Geometry check sheet. Reference: the model listing, model coordinates, mm. A direction names the side the tool comes from. Give positions to 0.01 mm unless a question says otherwise; leave off trailing zeros. Loops run counter-clockwise (first coordinate to the right, second up) from the corner with the lowest first, then second, coordinate; pieces in that order, holes last.
1. Tool access check on faces 4 (the cylindrical face through (28.276, 121.639, -3.057)), 5 (the flat face through (3.019, 170, -3)), 6 (the flat face through (14.548, 114.345, -3.057)). Record the directions out of +Z, -Z, +X, -X, +Y, -Y that give a thin tool (end or side, any length) a straight path to the whole face; none if there is none.
2. Cross-section at D-D, the plane y = 134. Record the cut outline in (x, z), plus the area to 3 significant figures.
3. Cross-section at A-A, the plane z = -4.75. Record the cut outline in (x, y).
4. Cross-section at B-B, the plane x = 18. Record the cut outline in (y, z).
5. Material ranges on L1, parallel to Y at x = 19.75, z = -4; L2, parallel to X at y = 184, z = -4.5; L3, parallel to Y at x = 6, z = -4, recorded low to high.
6. Go/stop test with flat-tipped pins: pin 1 Ø3 at (y, z) = (96, -3) entering from -X; pin 2 Ø1.9 at (y, z) = (171.5, -4) entering from +X. Record where each tip stops, or that it passes through.
7. Cross-section at C-C, the plane y = 95.5. Record the cut outline in (x, z).
8. Release check for a two-part mould opening along Y. For faces 1 (the flat face through (15.196, 113.191, -3.057)), 2 (the cylindrical face through (2.642, 133.722, -3.057)), 3 (the flat face through (3.019, 93, -3)) record: +Y half, -Y half, draft (parallel to the pull), parting line (faces both ways), or undercut.
from build123d import *

# Parameters (mm, degrees)
BOSS_EXTRUDE1_DEPTH = 6.2
SKETCH2_W           = 22.942955783
SKETCH2_H           = 33.63345143
CUT_EXTRUDE1_DEPTH  = 10
SKETCH3_W           = 6.2
SKETCH3_H           = 21.335576668
CUT_EXTRUDE2_DEPTH  = 10
SKETCH4_W           = 6.2
SKETCH4_H           = 34.092468675
CUT_EXTRUDE3_DEPTH  = 10


with BuildPart() as part:
    # Sketch1 → Boss-Extrude1 (new body)
    with BuildSketch(Plane.XY):
        with BuildLine():
            Line((5.938584497, 132.670572888), (23.853053602, 126.575547243))
            ThreePointArc((23.853053602, 126.575547243), (28.280634989, 121.537232872), (24.198169049, 116.215432378))
            Line((24.198169049, 116.215432378), (5.937692527, 110.081409755))
            ThreePointArc((5.937692527, 110.081409755), (3.69123593, 108.257803943), (3.019475766, 105.443404596))
            Line((3.019475766, 105.443404596), (3.019475766, 19.274702795))
            Line((3.019475766, 19.274702795), (1.719475766, 19.274702795))
            Line((1.719475766, 19.274702795), (1.719475766, 105.386747909))
            ThreePointArc((1.719475766, 105.386747909), (2.613791193, 108.9861771), (5.506131352, 111.307827159))
            Line((5.506131352, 111.307827159), (23.847136202, 117.468900696))
            ThreePointArc((23.847136202, 117.468900696), (26.980585626, 121.515340919), (23.543843406, 125.30756806))
            Line((23.543843406, 125.30756806), (5.504633735, 131.445034089))
            ThreePointArc((5.504633735, 131.445034089), (2.6133616, 133.766807499), (1.719475766, 137.365564846))
            Line((1.719475766, 137.365564846), (1.719475766, 223.477609961))
            Line((1.719475766, 223.477609961), (3.019475766, 223.477609961))
            Line((3.019475766, 223.477609961), (3.019475766, 137.30890816))
            ThreePointArc((3.019475766, 137.30890816), (3.691489205, 134.494106323), (5.938584497, 132.670572888))
        make_face()
    extrude(amount=-BOSS_EXTRUDE1_DEPTH)

    # Sketch2 → Cut-Extrude1 (cut)
    with BuildSketch(Plane.ZY.offset(-1.719475766)):
        with Locations((-7.178599834, 29.49715685)):
            Rectangle(SKETCH2_W, SKETCH2_H)
    extrude(amount=-CUT_EXTRUDE1_DEPTH, mode=Mode.SUBTRACT)

    # Sketch3 → Cut-Extrude2 (cut)
    with BuildSketch(Plane(origin=(3.019475766, 0, 0), x_dir=(0, 0, -1), z_dir=(1, 0, 0))):
        with Locations((3.1, 212.809821627)):
            Rectangle(SKETCH3_W, SKETCH3_H)
    extrude(amount=-CUT_EXTRUDE2_DEPTH, mode=Mode.SUBTRACT)

    # Sketch4 → Cut-Extrude3 (cut)
    with BuildSketch(Plane(origin=(3.019475766, 0, 0), x_dir=(0, 0, -1), z_dir=(1, 0, 0))):
        with Locations((3.1, 63.360116903)):
            Rectangle(SKETCH4_W, SKETCH4_H)
    extrude(amount=-CUT_EXTRUDE3_DEPTH, mode=Mode.SUBTRACT)


solid = part.part
Result:
1. face 4: +Z, -Z, +X
1. face 5: +Z, -Z, +X, +Y
1. face 6: +Z, -Z, -X
2. outline: (2.47, -6.2) - (4.05, -6.2) - (4.05, 0) - (2.47, 0) - close
2. area: 9.79 mm2
3. outline: (1.72, 80.41) - (3.02, 80.41) - (3.02, 105.44) arc R4.5 cw to (5.94, 110.08) - (24.2, 116.22) arc R5.28 ccw to (23.85, 126.58) - (5.94, 132.67) arc R4.5 cw to (3.02, 137.31) - (3.02, 202.14) - (1.72, 202.14) - (1.72, 137.37) arc R5.8 ccw to (5.5, 131.45) - (23.54, 125.31) arc R3.98 cw to (23.85, 117.47) - (5.51, 111.31) arc R5.8 ccw to (1.72, 105.39) - close
4. outline: (114.13, -6.2) - (115.5, -6.2) - (115.5, 0) - (114.13, 0) - close; (127.19, -6.2) - (128.57, -6.2) - (128.57, 0) - (127.19, 0) - close
5. L1: y = 114.72 to 116.09, 126.6 to 127.97
5. L2: x = 1.72 to 3.02
5. L3: y = 110.1 to 111.47, 131.28 to 132.65
6. pin 1: stops at x = 1.72
6. pin 2: stops at x = 3.02
7. outline: (1.72, -6.2) - (3.02, -6.2) - (3.02, 0) - (1.72, 0) - close
8. face 1: -Y half
8. face 2: undercut
8. face 3: draft
